Design review of the part built by this model. Coordinates are the model's own, in mm. Face numbers are marked on the shaded views. Give positions to 0.01 mm unless a question says otherwise; leave off trailing zeros. Order: outer loops, then holes, each group sorted by start corner. A loop starts at its lowest first (then second) coordinate and runs counter-clockwise, first axis right, second up. Notation, with made-up numbers: (39, 6) -> (70, 6) arc R17 cw to (70, 38) -> close; hole circle Ø6 at (70, 59.25). An arc over 180 degrees is marked (long way). Use a Markdown table: item, result. Add a question column.
```python
from build123d import *

# Parameters (mm, degrees)
F0_R          = 2.05
F0_R_2        = 20
F1_DEPTH      = 4
F2_R          = 1.95
F3_DEPTH      = 4
F4_SIZE       = 1
F5_R          = 23.05
F5_R_2        = 20
F6_DEPTH      = 10
F8_DEPTH      = 2
F9_R          = 0.8
F10_DEPTH     = 6
F11_SIZE      = 2
F12_T1_DEPTH  = 50
F12_T3_DEPTH  = 50
F12_T6_ANGLE  = 90
F12_T8_ANGLE  = 90
F12_T10_ANGLE = 90
F12_T12_ANGLE = 90


# Not quite as in the source:
# - a fillet or chamfer that OpenCascade refuses, or shapes differently, is made with other operations: its cross-section is extruded or revolved along the edge and cut away or added


with BuildPart() as f1:
    # F0 (on Front) → F1 (new body)
    with BuildSketch(Plane.XZ):
        with BuildLine():
            ThreePointArc((30, 25), (28.5355339059, 28.5355339059), (25, 30))
            Line((25, 30), (-25, 30))
            ThreePointArc((-25, 30), (-28.5355339059, 28.5355339059), (-30, 25))
            Line((-30, 25), (-30, -25))
            ThreePointArc((-30, -25), (-28.5355339059, -28.5355339059), (-25, -30))
            Line((-25, -30), (25, -30))
            ThreePointArc((25, -30), (28.5355339059, -28.5355339059), (30, -25))
            Line((30, -25), (30, 25))
        make_face()
        with Locations((-25, -25)):
            Circle(F0_R, mode=Mode.SUBTRACT)
        with Locations((25, -25)):
            Circle(F0_R, mode=Mode.SUBTRACT)
        Circle(F0_R_2, mode=Mode.SUBTRACT)
        with Locations((-25, 25)):
            Circle(F0_R, mode=Mode.SUBTRACT)
        with Locations((25, 25)):
            Circle(F0_R, mode=Mode.SUBTRACT)
    extrude(amount=F1_DEPTH)

    # F2 (on face) → F3 (join)
    with BuildSketch(Plane(origin=(0, 0, 0), x_dir=(-1, 0, 0), z_dir=(0, 1, 0))):
        with Locations((-19, 25)):
            Circle(F2_R)
        with Locations((19, 25)):
            Circle(F2_R)
        with Locations((19, -25)):
            Circle(F2_R)
        with Locations((-16, -25)):
            Circle(F2_R)
    extrude(amount=F3_DEPTH)

    # F4
    f4_edges = [f1.edges().sort_by_distance(p)[0] for p in [
        (17.95, 4, -25),
        (-17.05, 4, -25),
        (-17.05, 4, 25),
        (20.95, 4, 25),
    ]]
    chamfer(f4_edges, length=F4_SIZE)

    # F5 (on face) → F6 (join)
    with BuildSketch(Plane.XZ.offset(4)):
        Circle(F5_R)
        Circle(F5_R_2, mode=Mode.SUBTRACT)
    extrude(amount=F6_DEPTH)

    # F7 (on face) → F8 (cut)
    with BuildSketch(Plane(origin=(0, 0, 0), x_dir=(-1, 0, 0), z_dir=(0, 1, 0))):
        with BuildLine():
            ThreePointArc((13, -15.1986841536), (0, -20), (-13, -15.1986841536))
            Line((-13, -15.1986841536), (-13, -23))
            ThreePointArc((-13, -23), (-12.4142135624, -24.4142135624), (-11, -25))
            Line((-11, -25), (11, -25))
            ThreePointArc((11, -25), (12.4142135624, -24.4142135624), (13, -23))
            Line((13, -23), (13, -15.1986841536))
        make_face()
    extrude(amount=-F8_DEPTH, mode=Mode.SUBTRACT)

    # F9 (on face) → F10 (cut)
    with BuildSketch(Plane(origin=(0, -2, 0), x_dir=(-1, 0, 0), z_dir=(0, 1, 0))):
        with Locations((-11.4065121626, -18.2542352698)):
            Circle(F9_R)
        with Locations((11.4065121626, -18.2542352698)):
            Circle(F9_R)
    extrude(amount=-F10_DEPTH, mode=Mode.SUBTRACT)

    # F11
    f11_edges = [f1.edges().sort_by_distance(p)[0] for p in [
        (22.95, -4, 25),
        (-27.05, -4, 25),
        (-27.05, -4, -25),
        (22.95, -4, -25),
    ]]
    chamfer(f11_edges, length=F11_SIZE)

    # F12: chamfer of 1 on 8 edges, made by hand

    # F12_s2 → F12_t1 (cut)
    with BuildSketch(Plane.XY.offset(-25)):
        with BuildLine():
            Line((28.9717157288, -4.0282842712), (30.0282842712, -2.9717157288))
            Line((30.0282842712, -2.9717157288), (30.0482842712, -2.9717157288))
            ThreePointArc((30.0482842712, -2.9717157288), (30.02, -3.4858578644), (30.02, -4))
            Line((30.02, -4), (30, -4.02))
            ThreePointArc((30, -4.02), (29.4858578644, -4.02), (28.9717157288, -4.0482842712))
            Line((28.9717157288, -4.0482842712), (28.9717157288, -4.0282842712))
        make_face()
        with BuildLine():
            Line((-28.9717157288, -4.0282842712), (-30.0282842712, -2.9717157288))
            Line((-30.0282842712, -2.9717157288), (-30.0482842712, -2.9717157288))
            ThreePointArc((-30.0482842712, -2.9717157288), (-30.02, -3.4858578644), (-30.02, -4))
            Line((-30.02, -4), (-30, -4.02))
            ThreePointArc((-30, -4.02), (-29.4858578644, -4.02), (-28.9717157288, -4.0482842712))
            Line((-28.9717157288, -4.0482842712), (-28.9717157288, -4.0282842712))
        make_face()
    extrude(amount=F12_T1_DEPTH, mode=Mode.SUBTRACT)

    # F12_s4 → F12_t3 (cut)
    with BuildSketch(Plane.YZ.offset(-25)):
        with BuildLine():
            Line((-4.0282842712, 28.9717157288), (-2.9717157288, 30.0282842712))
            Line((-2.9717157288, 30.0282842712), (-2.9717157288, 30.0482842712))
            ThreePointArc((-2.9717157288, 30.0482842712), (-3.4858578644, 30.02), (-4, 30.02))
            Line((-4, 30.02), (-4.02, 30))
            ThreePointArc((-4.02, 30), (-4.02, 29.4858578644), (-4.0482842712, 28.9717157288))
            Line((-4.0482842712, 28.9717157288), (-4.0282842712, 28.9717157288))
        make_face()
        with BuildLine():
            Line((-4.0282842712, -28.9717157288), (-2.9717157288, -30.0282842712))
            Line((-2.9717157288, -30.0282842712), (-2.9717157288, -30.0482842712))
            ThreePointArc((-2.9717157288, -30.0482842712), (-3.4858578644, -30.02), (-4, -30.02))
            Line((-4, -30.02), (-4.02, -30))
            ThreePointArc((-4.02, -30), (-4.02, -29.4858578644), (-4.0482842712, -28.9717157288))
            Line((-4.0482842712, -28.9717157288), (-4.0282842712, -28.9717157288))
        make_face()
    extrude(amount=F12_T3_DEPTH, mode=Mode.SUBTRACT)

    # F12_s5 → F12_t6 (revolve, cut)
    with BuildSketch(Plane.XY.offset(25)):
        with BuildLine():
            Line((28.9717157288, -4.0282842712), (30.0282842712, -2.9717157288))
            Line((30.0282842712, -2.9717157288), (30.0482842712, -2.9717157288))
            ThreePointArc((30.0482842712, -2.9717157288), (30.02, -3.4858578644), (30.02, -4))
            Line((30.02, -4), (30, -4.02))
            ThreePointArc((30, -4.02), (29.4858578644, -4.02), (28.9717157288, -4.0482842712))
            Line((28.9717157288, -4.0482842712), (28.9717157288, -4.0282842712))
        make_face()
    revolve(axis=Axis((25, -4, 25), (0, -1, 0)), revolution_arc=F12_T6_ANGLE, mode=Mode.SUBTRACT)

    # F12_s7 → F12_t8 (revolve, cut)
    with BuildSketch(Plane.YZ.offset(-25)):
        with BuildLine():
            Line((-4.0282842712, 28.9717157288), (-2.9717157288, 30.0282842712))
            Line((-2.9717157288, 30.0282842712), (-2.9717157288, 30.0482842712))
            ThreePointArc((-2.9717157288, 30.0482842712), (-3.4858578644, 30.02), (-4, 30.02))
            Line((-4, 30.02), (-4.02, 30))
            ThreePointArc((-4.02, 30), (-4.02, 29.4858578644), (-4.0482842712, 28.9717157288))
            Line((-4.0482842712, 28.9717157288), (-4.0282842712, 28.9717157288))
        make_face()
    revolve(axis=Axis((-25, -4, 25), (0, -1, 0)), revolution_arc=F12_T8_ANGLE, mode=Mode.SUBTRACT)

    # F12_s9 → F12_t10 (revolve, cut)
    with BuildSketch(Plane.XY.offset(-25)):
        with BuildLine():
            Line((-28.9717157288, -4.0282842712), (-30.0282842712, -2.9717157288))
            Line((-30.0282842712, -2.9717157288), (-30.0482842712, -2.9717157288))
            ThreePointArc((-30.0482842712, -2.9717157288), (-30.02, -3.4858578644), (-30.02, -4))
            Line((-30.02, -4), (-30, -4.02))
            ThreePointArc((-30, -4.02), (-29.4858578644, -4.02), (-28.9717157288, -4.0482842712))
            Line((-28.9717157288, -4.0482842712), (-28.9717157288, -4.0282842712))
        make_face()
    revolve(axis=Axis((-25, -4, -25), (0, -1, 0)), revolution_arc=F12_T10_ANGLE, mode=Mode.SUBTRACT)

    # F12_s11 → F12_t12 (revolve, cut)
    with BuildSketch(Plane.YZ.offset(25)):
        with BuildLine():
            Line((-4.0282842712, -28.9717157288), (-2.9717157288, -30.0282842712))
            Line((-2.9717157288, -30.0282842712), (-2.9717157288, -30.0482842712))
            ThreePointArc((-2.9717157288, -30.0482842712), (-3.4858578644, -30.02), (-4, -30.02))
            Line((-4, -30.02), (-4.02, -30))
            ThreePointArc((-4.02, -30), (-4.02, -29.4858578644), (-4.0482842712, -28.9717157288))
            Line((-4.0482842712, -28.9717157288), (-4.0282842712, -28.9717157288))
        make_face()
    revolve(axis=Axis((25, -4, -25), (0, -1, 0)), revolution_arc=F12_T12_ANGLE, mode=Mode.SUBTRACT)


solid = f1.part
```
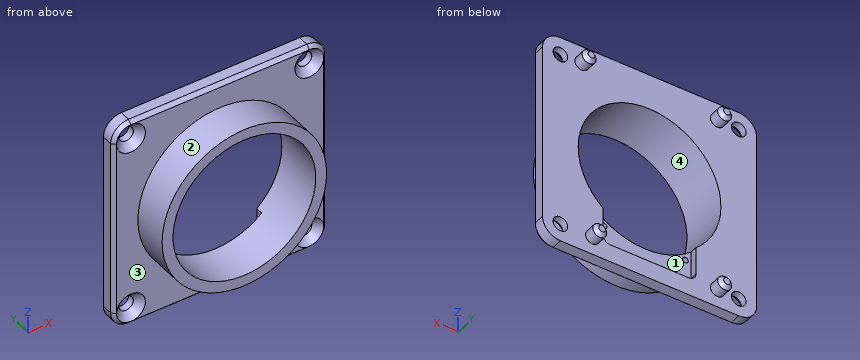
1) Add section D-D (x = 8). Give the boundary of the cut face in (y, z), then the cut area to 3 significant figures.
2) For L1, parallel to Z at x = -25, y = -1.2; L2, parallel to X at y = -3.25, z = 26.5; L3, parallel to X at y = -2.25, z = -0.5, list the stretches that pass through material, from the lowest coordinate up. Write a range as [from, to].
3) Add section A-A (x = 0). Give the boundary of the cut face in (y, z), then the cut area to 3 significant figures.
4) The part is to be moulded in two halves that separate along Z. For the marked faces 1, 2, 3 and 4, say which applies: +Z half, -Z half, draft (parallel to the pull), parting line (faces both ways), or undercut.
5) Insertion check: pin 1 (8 mm diameter, centred on x = -15.5, y = -9.5, fed in from +Z); pin 2 (1 mm diameter, centred on x = -2.5, y = -6.5, fed in from +Z); pin 3 (6 mm diameter, centred on y = -11, z = 11.5, fed in from +X); pin 4 (3.5 mm diameter, centred on x = -25, z = 25, fed in from -Y). Each pin has a flat end and moves straight along its axis. Give the tip position at first contact, or say it passes through.
6) Add section C-C (z = -13.5). Give the boundary of the cut face in (x, y).
7) Add section B-B (z = 0). Give the boundary of the cut face in (x, y).
Worked answers:
| question | item | result |
|---|---|---|
| 1 | outline | (-14, -21.62) -> (-4, -21.62) -> (-4, -29) -> (-3, -30) -> (0, -30) -> (0, -25) -> (-2, -25) -> (-2, -18.33) -> (-14, -18.33) -> close; (-14, 18.33) -> (0, 18.33) -> (0, 30) -> (-3, 30) -> (-4, 29) -> (-4, 21.62) -> (-14, 21.62) -> close |
| 1 | area | 145 mm^2 |
| 2 | L1 | [-30, -27.05], [-22.95, 22.95], [27.05, 30] |
| 2 | L2 | [-29.51, -27.94], [-22.06, 22.06], [27.94, 29.51] |
| 2 | L3 | [-30, -19.99], [19.99, 30] |
| 3 | outline | (-14, -23.05) -> (-4, -23.05) -> (-4, -29) -> (-3, -30) -> (0, -30) -> (0, -25) -> (-2, -25) -> (-2, -20) -> (-14, -20) -> close; (-14, 20) -> (0, 20) -> (0, 30) -> (-3, 30) -> (-4, 29) -> (-4, 23.05) -> (-14, 23.05) -> close |
| 3 | area | 130 mm^2 |
| 4 | face 1 | undercut |
| 4 | face 2 | parting line |
| 4 | face 3 | draft |
| 4 | face 4 | undercut |
| 5 | pin 1 | z = 19.98 |
| 5 | pin 2 | z = 22.96 |
| 5 | pin 3 | x = 21.43 |
| 5 | pin 4 | through |
| 6 | outline | (-30, -3) -> (-29, -4) -> (-18.68, -4) -> (-18.68, -14) -> (-14.76, -14) -> (-14.76, 0) -> (-30, 0) -> close; (14.76, -14) -> (18.68, -14) -> (18.68, -4) -> (29, -4) -> (30, -3) -> (30, 0) -> (14.76, 0) -> close |
| 7 | outline | (-30, -3) -> (-29, -4) -> (-23.05, -4) -> (-23.05, -14) -> (-20, -14) -> (-20, 0) -> (-30, 0) -> close; (20, -14) -> (23.05, -14) -> (23.05, -4) -> (29, -4) -> (30, -3) -> (30, 0) -> (20, 0) -> close |
